```python
from build123d import *

# Parameters (mm, degrees)
BOSS_EXTRUDE1_DEPTH = 15.24
CHAMFER1_SIZE       = 9
FILLET1_R           = 20
SKETCH2_R           = 2.38125
CUT_EXTRUDE1_DEPTH  = 15.24


with BuildPart() as part:
    # Sketch1 → Boss-Extrude1 (new body)
    with BuildSketch(Plane(origin=(0, 0, 0), x_dir=(1, 0, 0), z_dir=(0, 1, 0))):
        Polygon((-365.243004426, 189.912666736), (135.648161339, 189.912666736), (271.202578456, 104.912666736), (431.972487964, 104.912666736), (471.202578456, 89.912666736), (471.202578456, 9.912666736), (431.972487964, -5.087333264), (271.202578456, -5.087333264), (135.648161339, -90.087333264), (-365.243004426, -90.087333264), (-500.797421544, -5.087333264), (-661.567331052, -5.087333264), (-700.797421544, 9.912666736), (-700.797421544, 89.912666736), (-661.567331052, 104.912666736), (-500.797421544, 104.912666736), align=None)
    extrude(amount=BOSS_EXTRUDE1_DEPTH)

    # Chamfer1
    chamfer1_edges = [part.edges().sort_by_distance(p)[0] for p in [
        (451.58753321, 15.24, -2.412666736),
        (471.202578456, 15.24, -49.912666736),
        (451.58753321, 15.24, -97.412666736),
        (351.58753321, 15.24, -104.912666736),
        (203.425369898, 15.24, -147.412666736),
        (-114.797421544, 15.24, -189.912666736),
        (-433.020212985, 15.24, -147.412666736),
        (-581.182376298, 15.24, -104.912666736),
        (-681.182376298, 15.24, -97.412666736),
        (-700.797421544, 15.24, -49.912666736),
        (203.425369898, 15.24, 47.587333264),
        (-681.182376298, 15.24, -2.412666736),
        (-581.182376298, 15.24, 5.087333264),
        (-433.020212985, 15.24, 47.587333264),
        (-114.797421544, 15.24, 90.087333264),
        (351.58753321, 15.24, 5.087333264),
    ]]
    chamfer(chamfer1_edges, length=CHAMFER1_SIZE)

    # Fillet1
    fillet1_edges = [part.edges().sort_by_distance(p)[0] for p in [
        (269.908400539, 10.74, 0.587333264),
        (-499.503243626, 10.74, 0.587333264),
        (269.908400539, 10.74, -100.412666736),
        (-499.503243626, 10.74, -100.412666736),
    ]]
    fillet(fillet1_edges, radius=FILLET1_R)

    # Sketch2 → Cut-Extrude1 (cut)
    with BuildSketch(Plane.XZ):
        with BuildLine():
            ThreePointArc((-628.416171544, -70.550166736), (-629.113623521, -68.866368714), (-630.797421544, -68.168916736))
            Line((-630.797421544, -68.168916736), (-630.797421544, -70.550166736))
            Line((-630.797421544, -70.550166736), (-628.416171544, -70.550166736))
        make_face()
        with BuildLine():
            Line((-630.797421544, -70.550166736), (-630.797421544, -68.168916736))
            ThreePointArc((-630.797421544, -68.168916736), (-632.481219566, -72.233964759), (-628.416171544, -70.550166736))
            Line((-628.416171544, -70.550166736), (-630.797421544, -70.550166736))
        make_face()
        with BuildLine():
            Line((-630.797421544, -31.656416736), (-630.797421544, -29.275166736))
            Line((-630.797421544, -29.275166736), (-628.416171544, -29.275166736))
            ThreePointArc((-628.416171544, -29.275166736), (-632.481219566, -27.591368714), (-630.797421544, -31.656416736))
        make_face()
        with BuildLine():
            Line((-628.416171544, -29.275166736), (-630.797421544, -29.275166736))
            Line((-630.797421544, -29.275166736), (-630.797421544, -31.656416736))
            ThreePointArc((-630.797421544, -31.656416736), (-629.113623521, -30.958964759), (-628.416171544, -29.275166736))
        make_face()
        with BuildLine():
            ThreePointArc((-564.916171544, -29.275166736), (-567.297421544, -26.893916736), (-569.678671544, -29.275166736))
            Line((-569.678671544, -29.275166736), (-567.297421544, -29.275166736))
            Line((-567.297421544, -29.275166736), (-567.297421544, -31.656416736))
            ThreePointArc((-567.297421544, -31.656416736), (-565.613623521, -30.958964759), (-564.916171544, -29.275166736))
        make_face()
        with BuildLine():
            Line((-567.297421544, -29.275166736), (-569.678671544, -29.275166736))
            ThreePointArc((-569.678671544, -29.275166736), (-568.981219566, -30.958964759), (-567.297421544, -31.656416736))
            Line((-567.297421544, -31.656416736), (-567.297421544, -29.275166736))
        make_face()
        with BuildLine():
            ThreePointArc((-564.916171544, -70.550166736), (-565.613623521, -68.866368714), (-567.297421544, -68.168916736))
            Line((-567.297421544, -68.168916736), (-567.297421544, -70.550166736))
            Line((-567.297421544, -70.550166736), (-569.678671544, -70.550166736))
            ThreePointArc((-569.678671544, -70.550166736), (-567.297421544, -72.931416736), (-564.916171544, -70.550166736))
        make_face()
        with BuildLine():
            Line((-567.297421544, -70.550166736), (-567.297421544, -68.168916736))
            ThreePointArc((-567.297421544, -68.168916736), (-568.981219566, -68.866368714), (-569.678671544, -70.550166736))
            Line((-569.678671544, -70.550166736), (-567.297421544, -70.550166736))
        make_face()
        with Locations(Location((337.702578456, -70.550166736, 0), (0, 0, 270))):
            Circle(SKETCH2_R)
        with Locations(Location((337.702578456, -29.275166736, 0), (0, 0, 270))):
            Circle(SKETCH2_R)
        with Locations(Location((401.202578456, -29.275166736, 0), (0, 0, 270))):
            Circle(SKETCH2_R)
        with Locations(Location((401.202578456, -70.550166736, 0), (0, 0, 270))):
            Circle(SKETCH2_R)
    extrude(amount=-CUT_EXTRUDE1_DEPTH, mode=Mode.SUBTRACT)


solid = part.part
```
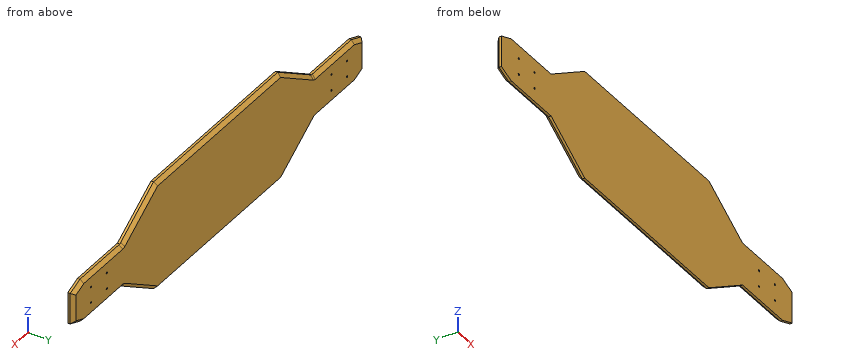
CAD build for the part. Positions are in the model's coordinates, mm. Round coordinates to 2 decimals unless told otherwise and drop trailing zeros. Order: outer loops, then holes, each group sorted by start corner. A loop starts at its lowest first (then second) coordinate and runs counter-clockwise, first axis right, second up.
Q1. Slice it at A-A (x = -597). Write the cut outline in (y, z), and give its area (3 significant figures).
Q2. Drop flat-ended pins along their axis: pin 1 (4.5 mm diameter, centred on x = 401.2, z = -29.28, fed in from +Y); pin 2 (3 mm diameter, centred on y = 11, z = 20, fed in from +X); pin 3 (3 mm diameter, centred on x = -459, y = 9.5, fed in from +Z); pin 4 (3.5 mm diameter, centred on x = 373, y = 4.5, fed in from -Z). Give the stop position or say it passes through.
Q3. Slice it at C-C (z = -135). Write the cut outline in (x, y).
Q4. Slice it at B-B (y = 11.5). State how many separate pieces and enclosed holes the cut face has, and give its area (3 significant figures).
Q5. Wall check: L1, parallel to X at y = 13, z = -70.5; L2, parallel to Z at x = -643, y = 1.5; L3, parallel to X at y = 4.25, z = 28. Give the ranges that are in metal, low to high.
Results below:
1. outline: (0, -104.91) - (6.24, -104.91) - (15.24, -95.91) - (15.24, -3.91) - (6.24, 5.09) - (0, 5.09) - close
1. area: 1,600 mm2
2. pin 1: passes through
2. pin 2: stops at x = 242.16
2. pin 3: stops at z = 29.45
2. pin 4: stops at z = -104.91
3. outline: (-452.82, 0) - (223.22, 0) - (223.22, 6.24) - (206.28, 15.24) - (-435.87, 15.24) - (-452.82, 6.24) - close
4. separate pieces: 1
4. enclosed holes: 8
4. area: 222,000 mm2
5. L1: x = -694.04 to -633.18, -628.42 to -569.68, -564.92 to 335.32, 340.08 to 398.82, 403.58 to 464.44
5. L2: z = -104.91 to 5.09
5. L3: x = -464.26 to 234.66
